from build123d import *

# Parameters (mm, degrees)
SKETCH1_R           = 50
SKETCH1_R_2         = 44
BOSS_EXTRUDE1_DEPTH = 4
SKETCH2_R           = 10
BOSS_EXTRUDE2_DEPTH = 5
SKETCH3_W           = 5
SKETCH3_H           = 36
BOSS_EXTRUDE3_DEPTH = 2
SKETCH4_R           = 2.5
CUT_EXTRUDE1_DEPTH  = 6
CIRPATTERN1_COUNT   = 6


with BuildPart() as part:
    # Sketch1 → Boss-Extrude1 (new, symmetric)
    with BuildSketch(Plane.XY):
        Circle(SKETCH1_R)
        Circle(SKETCH1_R_2, mode=Mode.SUBTRACT)
    extrude(amount=BOSS_EXTRUDE1_DEPTH, both=True)



with BuildPart() as body_2:
    # Sketch2 → Boss-Extrude2 (new, symmetric)
    with BuildSketch(Plane.XY):
        Circle(SKETCH2_R)
    extrude(amount=BOSS_EXTRUDE2_DEPTH, both=True)


with BuildPart() as part_1:
    add(part.part)

    add(body_2.part)  # Boss-Extrude3 merges body 2
    # Sketch3 → Boss-Extrude3 (add, symmetric)
    with BuildSketch(Plane.XY):
        with Locations((0, 27)):
            Rectangle(SKETCH3_W, SKETCH3_H)
    boss_extrude3 = extrude(amount=BOSS_EXTRUDE3_DEPTH, both=True)

    # Sketch4 → Cut-Extrude1 (cut, symmetric)
    with BuildSketch(Plane.XY):
        Circle(SKETCH4_R)
    extrude(amount=CUT_EXTRUDE1_DEPTH, both=True, mode=Mode.SUBTRACT)

    # CirPattern1: Boss-Extrude3 ×6 about axis
    cirpattern1_axis = Axis((0, 0, 0), (0, 0, 1))
    for i in range(1, CIRPATTERN1_COUNT):
        add(boss_extrude3.rotate(cirpattern1_axis, i * 360 / CIRPATTERN1_COUNT))


solid = part_1.part
The listing builds one solid part. Answer for the finished solid, in the listing's coordinates (mm). A direction names the side the tool comes from. Round coordinates to 2 decimals unless told otherwise and drop trailing zeros. Write each loop counter-clockwise with the first axis right and the second up, starting at its lowest first coordinate (ties: lowest second). Pieces come first, ordered by that corner, then holes. Notation, with made-up numbers: (-21.5, -21.75) - (-7.5, -21.75) arc R30 cw to (-7.5, 3.25) - close; hole circle Ø11 at (-33.5, -36). An arc over 180 degrees is marked (long way). Use a Markdown table: item, result. Add a question column.
1. The part is cut by section B-B (x = 0). Write down the section's boundary in (y, z).
2. The part is cut by section C-C (z = 0). Write down the section's boundary in (x, y), and give its area (3 significant figures).
3. For a pull along X with two mould halves and no side action, classify faces 1 (the face through (-23, -14, 2)), 2 (the face through (2, -2, -5)), 3 (the face through (-2.5, 27, 0)) as +X half, -X half, draft (parallel to the pull), parting line (faces both ways), or undercut.
4. Flat-ended cylindrical pins translate along their axes: P1, Ø5.5, axis at x = 0, y = -22, coming from the -Z side; P2, Ø4.5, axis at y = -34, z = 1, coming from the -X side; P3, Ø1, axis at x = 14.5, z = -3.5, coming from the -Y side; P4, Ø10, axis at x = 12.5, y = 19.5, coming from the -Z side. Find the tip coordinate at first contact, or state that the pin passes through.
5. The part is cut by section A-A (y = 0). Write down the section's boundary in (x, z), and give its area (3 significant figures).
6. A tool of negligible diameter and unlimited length cuts with its end or side. For faces 4 (the face through (2, -2, 5)), 5 (the face through (0, -27, -2)), 6 (the face through (0, -27, 2)), 7 (the face through (21.76, 15.45, 0.03)), from which of +Z, -Z, +X, -X, +Y, -Y can it reach the whole face along a straight path? Write none if from no direction.
7. The part is cut by section D-D (y = -14). Write down the section's boundary in (x, z), and give its area (3 significant figures).
8. Consider line 1 (Y direction, x = 0, z = 2.25); line 2 (Y direction, x = 0, z = 0); line 3 (Y direction, x = -6, z = 1). Determine where each line is inside the solid, lowest interval first.
Reported:
| question | item | result |
|---|---|---|
| 1 | outline | (-50, -4) - (-44, -4) - (-44, -2) - (-10, -2) - (-10, -5) - (-2.5, -5) - (-2.5, 5) - (-10, 5) - (-10, 2) - (-44, 2) - (-44, 4) - (-50, 4) - close; (2.5, -5) - (10, -5) - (10, -2) - (44, -2) - (44, -4) - (50, -4) - (50, 4) - (44, 4) - (44, 2) - (10, 2) - (10, 5) - (2.5, 5) - close |
| 2 | outline | circle Ø100 at (0, 0); hole (-39.29, -19.8) - (-9.64, -2.68) arc R10 cw to (-9.64, 2.68) - (-39.29, 19.8) arc R44 ccw to start; hole (-36.79, -24.13) arc R44 ccw to (-2.5, -43.93) - (-2.5, -9.68) arc R10 cw to (-7.14, -7.01) - close; hole (-36.79, 24.13) - (-7.14, 7.01) arc R10 cw to (-2.5, 9.68) - (-2.5, 43.93) arc R44 ccw to start; hole circle Ø5 at (0, 0); hole (2.5, -43.93) arc R44 ccw to (36.79, -24.13) - (7.14, -7.01) arc R10 cw to (2.5, -9.68) - close; hole (2.5, 9.68) arc R10 cw to (7.14, 7.01) - (36.79, 24.13) arc R44 ccw to (2.5, 43.93) - close; hole (9.64, -2.68) - (39.29, -19.8) arc R44 ccw to (39.29, 19.8) - (9.64, 2.68) arc R10 cw to start |
| 2 | area | 3,090 mm^2 |
| 3 | face 1 | undercut |
| 3 | face 2 | draft |
| 3 | face 3 | undercut |
| 4 | P1 | z = -2 |
| 4 | P2 | x = -38.63 |
| 4 | P3 | y = -48 |
| 4 | P4 | through |
| 5 | outline | (-50, -4) - (-44, -4) - (-44, 4) - (-50, 4) - close; (-10, -5) - (-2.5, -5) - (-2.5, 5) - (-10, 5) - close; (2.5, -5) - (10, -5) - (10, 5) - (2.5, 5) - close; (44, -4) - (50, -4) - (50, 4) - (44, 4) - close |
| 5 | area | 246 mm^2 |
| 6 | face 4 | +Z, +X, -X, +Y, -Y |
| 6 | face 5 | -Z |
| 6 | face 6 | +Z |
| 6 | face 7 | +Z, -Z |
| 7 | outline | (-48, -4) - (-41.71, -4) - (-41.71, 4) - (-48, 4) - close; (-29.25, -2) - (-19.25, -2) - (-19.25, 2) - (-29.25, 2) - close; (-2.5, -2) - (2.5, -2) - (2.5, 2) - (-2.5, 2) - close; (19.25, -2) - (29.25, -2) - (29.25, 2) - (19.25, 2) - close; (41.71, -4) - (48, -4) - (48, 4) - (41.71, 4) - close |
| 7 | area | 201 mm^2 |
| 8 | line 1 | -50 to -44, -10 to -2.5, 2.5 to 10, 44 to 50 |
| 8 | line 2 | -50 to -2.5, 2.5 to 50 |
| 8 | line 3 | -49.64 to -43.59, -8 to 8, 43.59 to 49.64 |
